Input: part model. Units: mm. Frame: model coordinates. A direction names the side the tool comes from. Coordinates: 2 decimals unless noted, no trailing zeros. Order: outer loops, then holes, each group sorted by start corner. A loop starts at its lowest first (then second) coordinate and runs counter-clockwise, first axis right, second up. Notation, with made-up numbers: M 26,23.25 L 65,23.25 A30 ccw 65,51.25 Z; hole C 43,64 d10. An arc over 180 degrees is marked long. Answer in a Markdown table with one row per item.
from build123d import *

# Parameters (mm, degrees)
F1_DEPTH = 2
F2_DEPTH = 3
F3_DEPTH = 3


# Not quite as in the source:
# - a feature names something its author has since deleted; it is built from what else it names


with BuildPart() as f1:
    # F0 (on Top) → F1 (new body)
    with BuildSketch(Plane.XY):
        Polygon((-43.2085677565, 22.6745967576), (-58.8549531333, -4.4257376699), (-38.4300476107, -4.4257376699), (-40.2088151152, 5.6621541398), (-48.0090622621, 5.6621541398), (-48.5864125313, 6.6621541398), (-48.0090622621, 7.6621541398), (-40.5614690766, 7.6621541398), align=None)
    extrude(amount=F1_DEPTH)



with BuildPart() as f1b:
    # F0 (on Top) → F1, piece 2 (new body)
    with BuildSketch(Plane.XY):
        Polygon((-41.2085677565, 22.6745967576), (-36.4300476107, -4.4257376699), (-25.5239465254, -4.4257376699), (-23.5239465254, -4.4257376699), (-23.1770010553, -4.4257376699), (-25.5239465254, 8.8844515061), (-33.4898163741, 8.8844515061), (-34.0671666433, 9.8844515061), (-33.4898163741, 10.8844515061), (-22.7936475677, 10.8844515061), (-20.0940481363, -4.4257376699), (-3.2846095154, -4.4257376699), (4.538583173, 9.1244295439), (-3.2846095154, 22.6745967576), (-20.0940481363, 22.6745967576), (-24.4790815038, 15.0794961721), (-25.6024042349, 14.7936511306), (-33.2868439501, 22.6745967576), align=None)
        Polygon((-15.4996355878, 9.1244295439), (-13.5944822068, 12.424251996), (-9.7841754448, 12.424251996), (-7.8790220638, 9.1244295439), (-9.7841754448, 5.8246070917), (-13.5944822068, 5.8246070917), align=None, mode=Mode.SUBTRACT)
    extrude(amount=F1_DEPTH)


with BuildPart() as f1_1:
    add(f1.part)

    add(f1b.part)  # F2 merges F1b
    # F0 (on Top) → F2 (join)
    with BuildSketch(Plane.XY):
        Polygon((-2.8602079346, 24.6745967576), (-44.3632682949, 24.6745967576), (-62.3190547484, -6.4257376699), (-38.9180315569, -6.4257376699), (-2.129908977, -6.4257376699), (6.8479842498, 9.1244295439), (15.8258774766, 24.6745967576), align=None)
        Polygon((-38.4300476107, -4.4257376699), (-58.8549531333, -4.4257376699), (-43.2085677565, 22.6745967576), (-41.2085677565, 22.6745967576), (-33.2868439501, 22.6745967576), (-30.5356123181, 22.6745967576), (-20.0940481363, 22.6745967576), (-3.2846095154, 22.6745967576), (4.538583173, 9.1244295439), (-3.2846095154, -4.4257376699), (-20.0940481363, -4.4257376699), (-23.1770010553, -4.4257376699), (-23.5239465254, -4.4257376699), (-25.5239465254, -4.4257376699), (-36.4300476107, -4.4257376699), align=None, mode=Mode.SUBTRACT)
        Polygon((12.3617758614, 22.6745967576), (5.6932837114, 11.1244295439), (-0.9752084386, 22.6745967576), align=None, mode=Mode.SUBTRACT)
        Polygon((-25.5239465254, 8.8844515061), (-23.1770010553, -4.4257376699), (-20.0940481363, -4.4257376699), (-22.7936475677, 10.8844515061), (-33.4898163741, 10.8844515061), (-34.0671666433, 9.8844515061), (-33.4898163741, 8.8844515061), align=None)
        Polygon((-40.2088151152, 5.6621541398), (-38.4300476107, -4.4257376699), (-36.4300476107, -4.4257376699), (-41.2085677565, 22.6745967576), (-43.2085677565, 22.6745967576), (-40.5614690766, 7.6621541398), align=None)
        Polygon((-20.0940481363, 22.6745967576), (-30.5356123181, 22.6745967576), (-24.1704509766, 16.1898996279), (-24.4790815038, 15.0794961721), align=None)
        Polygon((-30.5356123181, 22.6745967576), (-33.2868439501, 22.6745967576), (-25.6024042349, 14.7936511306), (-24.4790815038, 15.0794961721), (-24.1704509766, 16.1898996279), align=None)
        Polygon((-48.0090622621, 5.6621541398), (-40.2088151152, 5.6621541398), (-40.5614690766, 7.6621541398), (-48.0090622621, 7.6621541398), (-48.5864125313, 6.6621541398), align=None)
    extrude(amount=F2_DEPTH)

    # F0 (on Top) → F3 (join)
    with BuildSketch(Plane.XY):
        Polygon((-9.7841754448, 12.424251996), (-13.5944822068, 12.424251996), (-15.4996355878, 9.1244295439), (-13.5944822068, 5.8246070917), (-9.7841754448, 5.8246070917), (-7.8790220638, 9.1244295439), align=None)
    extrude(amount=F3_DEPTH)


solid = f1_1.part
1) Material intervals for probe 1 along Y at (x, z) = (-45, 2.2); probe 2 along Y at (x, z) = (-46.5, 2.85); probe 3 along Z at (x, y) = (-47.5, 9.5), sorted ascending.
Resolved:
| item | result |
|---|---|
| probe 1 | y = -6.43 to -4.43, 5.66 to 7.66, 19.57 to 23.57 |
| probe 2 | y = -6.43 to -4.43, 5.66 to 7.66, 16.97 to 20.97 |
| probe 3 | z = 0 to 2 |
2) Cut plane C-C, the plane x = -51. Output: boundary loops of the cut face in (y, z).
Resolved:
| item | result |
|---|---|
| outline | M -6.43,0 L 13.18,0 L 13.18,3 L 9.18,3 L 9.18,2 L -4.43,2 L -4.43,3 L -6.43,3 Z |
3) Contact query for flat-ended pins moving along their axis: pin 1 (0.5 mm diameter, centred on x = -45, z = 2.5, fed in from +Y); pin 2 (8 mm diameter, centred on x = -17, y = 3, fed in from +Z); pin 3 (1.1 mm diameter, centred on x = -48.5, z = 2.5, fed in from +Y). Output: stop coordinate, or through.
Resolved:
| item | result |
|---|---|
| pin 1 | stops at y = 24 |
| pin 2 | stops at z = 2 |
| pin 3 | stops at y = 18.46 |
4) Cut plane A-A, the plane z = 1.1. Output: boundary loops of the cut face in (x, y), and give its area (3 significant figures).
Resolved:
| item | result |
|---|---|
| outline | M -62.32,-6.43 L -2.13,-6.43 L 15.83,24.67 L -44.36,24.67 Z; hole M -0.98,22.67 L 5.69,11.12 L 12.36,22.67 Z |
| area | 1,790 mm2 |
5) Cut plane B-B, the plane y = 4. Output: boundary loops of the cut face in (x, z), and give its area (3 significant figures).
Resolved:
| item | result |
|---|---|
| outline | M -56.3,0 L 3.89,0 L 3.89,3 L 1.58,3 L 1.58,2 L -21.58,2 L -21.58,3 L -24.66,3 L -24.66,2 L -37.92,2 L -37.92,3 L -39.92,3 L -39.92,2 L -53.99,2 L -53.99,3 L -56.3,3 Z |
| area | 130 mm2 |
6) Reachability of faces 1 (the face through (-26, 10, 3)), 2 (the face through (-51.141, 8.935, 2.493)), 3 (the face through (9.074, 16.98, 1.479)) from +Z, -Z, +X, -X, +Y, -Y: full face, straight path, thin tool, end or side. Return the list, or none.
Resolved:
| item | result |
|---|---|
| face 1 | +Z, +X, -X, +Y, -Y |
| face 2 | +Z |
| face 3 | +Z, -Z |
7) Mould query, pull axis Y, two halves, no side actions, for faces 4 (the face through (-33, -6.426, 1)), 5 (the face through (-12, 9, 3)), 6 (the face through (2.406, 16.819, 1.479)), 7 (the face through (-41.904, 15.273, 2.493)). Classes: +Y half, -Y half, draft (parallel to the pull), parting line (faces both ways), or undercut.
Resolved:
| item | result |
|---|---|
| face 4 | -Y half |
| face 5 | draft |
| face 6 | undercut |
| face 7 | undercut |
